from build123d import *

# Parameters (mm, degrees)
SKETCH1_R            = 34.29
BOSS_EXTRUDE1_DEPTH  = 10.16
SKETCH2_R            = 33.02
CUT_EXTRUDE1_DEPTH   = 7.62
SKETCH3_R            = 3.81
BOSS_EXTRUDE2_DEPTH  = 1.27
CUT_EXTRUDE3_REACH   = 51.088
CUT_EXTRUDE4_REACH   = 51.088
CUT_EXTRUDE5_REACH   = 51.546
SKETCH11_R           = 2.032
M2_CLEARANCE_HOLE1_D = 2.4


with BuildPart() as part:
    # Sketch1 → Boss-Extrude1 (new body)
    with BuildSketch(Plane(origin=(0, 0, 0), x_dir=(1, 0, 0), z_dir=(0, 1, 0))):
        with Locations(Location((0, 0, 0), (0, 0, 270))):
            Circle(SKETCH1_R)
    extrude(amount=BOSS_EXTRUDE1_DEPTH)

    # Sketch2 → Cut-Extrude1 (cut)
    with BuildSketch(Plane(origin=(0, 10.16, 0), x_dir=(1, 0, 0), z_dir=(0, 1, 0))):
        with Locations(Location((0, 0, 0), (0, 0, 270))):
            Circle(SKETCH2_R)
    extrude(amount=-CUT_EXTRUDE1_DEPTH, mode=Mode.SUBTRACT)

    # Sketch3 → Boss-Extrude2 (add)
    with BuildSketch(Plane(origin=(0, 2.54, 0), x_dir=(1, 0, 0), z_dir=(0, 1, 0))):
        with Locations(Location((0, -15.24, 0), (0, 0, 270))):
            Circle(SKETCH3_R)
        with Locations(Location((0, 15.24, 0), (0, 0, 270))):
            Circle(SKETCH3_R)
    extrude(amount=BOSS_EXTRUDE2_DEPTH)

    # Sketch8 → Cut-Extrude3 (cut, up to next)
    with BuildSketch(Plane(origin=(0, 2.54, 0), x_dir=(1, 0, 0), z_dir=(0, 1, 0)), mode=Mode.PRIVATE) as cut_extrude3_sk1:
        with BuildLine():
            Line((3.683, 2.032), (-3.683, 2.032))
            ThreePointArc((-3.683, 2.032), (-4.581025612, 1.660025612), (-4.953, 0.762))
            Line((-4.953, 0.762), (-4.953, -0.762))
            ThreePointArc((-4.953, -0.762), (-4.581025612, -1.660025612), (-3.683, -2.032))
            Line((-3.683, -2.032), (3.683, -2.032))
            ThreePointArc((3.683, -2.032), (4.581025612, -1.660025612), (4.953, -0.762))
            Line((4.953, -0.762), (4.953, 0.762))
            ThreePointArc((4.953, 0.762), (4.581025612, 1.660025612), (3.683, 2.032))
        make_face()
    cut_extrude3_tool1 = extrude(cut_extrude3_sk1.sketch, amount=-CUT_EXTRUDE3_REACH, mode=Mode.PRIVATE) & part.part
    add(cut_extrude3_tool1.solids().sort_by_distance((0, 2.54, 0))[0], mode=Mode.SUBTRACT)

    # Sketch9 → Cut-Extrude4 (cut, up to next)
    with BuildSketch(Plane(origin=(0, 2.54, 0), x_dir=(1, 0, 0), z_dir=(0, 1, 0)), mode=Mode.PRIVATE) as cut_extrude4_sk1:
        with BuildLine():
            Line((-12.192, 0), (-9.144, 0))
            ThreePointArc((-9.144, 0), (-8.245974388, 0.371974388), (-7.874, 1.27))
            Line((-7.874, 1.27), (-7.874, 18.796))
            ThreePointArc((-7.874, 18.796), (-8.245974388, 19.694025612), (-9.144, 20.066))
            Line((-9.144, 20.066), (-12.192, 20.066))
            ThreePointArc((-12.192, 20.066), (-13.090025612, 19.694025612), (-13.462, 18.796))
            Line((-13.462, 18.796), (-13.462, 1.27))
            ThreePointArc((-13.462, 1.27), (-13.090025612, 0.371974388), (-12.192, 0))
        make_face()
    cut_extrude4_tool1 = extrude(cut_extrude4_sk1.sketch, amount=-CUT_EXTRUDE4_REACH, mode=Mode.PRIVATE) & part.part
    add(cut_extrude4_tool1.solids().sort_by_distance((-10.668, 2.54, -10.033))[0], mode=Mode.SUBTRACT)

    # Sketch11 → Cut-Extrude5 (cut, up to next)
    with BuildSketch(Plane.XZ, mode=Mode.PRIVATE) as cut_extrude5_sk1:
        with Locations(Location((15.875, 13.843, 0), (0, 0, 270))):
            Circle(SKETCH11_R)
    cut_extrude5_tool1 = extrude(cut_extrude5_sk1.sketch, amount=-CUT_EXTRUDE5_REACH, mode=Mode.PRIVATE) & part.part
    # Sketch11 → Cut-Extrude5 (cut, up to next)
    with BuildSketch(Plane.XZ, mode=Mode.PRIVATE) as cut_extrude5_sk2:
        with Locations(Location((-15.875, 13.843, 0), (0, 0, 270))):
            Circle(SKETCH11_R)
    cut_extrude5_tool2 = extrude(cut_extrude5_sk2.sketch, amount=-CUT_EXTRUDE5_REACH, mode=Mode.PRIVATE) & part.part
    # Sketch11 → Cut-Extrude5 (cut, up to next)
    with BuildSketch(Plane.XZ, mode=Mode.PRIVATE) as cut_extrude5_sk3:
        with Locations(Location((-15.875, -24.257, 0), (0, 0, 270))):
            Circle(SKETCH11_R)
    cut_extrude5_tool3 = extrude(cut_extrude5_sk3.sketch, amount=-CUT_EXTRUDE5_REACH, mode=Mode.PRIVATE) & part.part
    # Sketch11 → Cut-Extrude5 (cut, up to next)
    with BuildSketch(Plane.XZ, mode=Mode.PRIVATE) as cut_extrude5_sk4:
        with Locations(Location((15.875, -24.257, 0), (0, 0, 270))):
            Circle(SKETCH11_R)
    cut_extrude5_tool4 = extrude(cut_extrude5_sk4.sketch, amount=-CUT_EXTRUDE5_REACH, mode=Mode.PRIVATE) & part.part
    add(cut_extrude5_tool1.solids().sort_by_distance((15.875, 0, 13.843))[0], mode=Mode.SUBTRACT)
    add(cut_extrude5_tool2.solids().sort_by_distance((-15.875, 0, 13.843))[0], mode=Mode.SUBTRACT)
    add(cut_extrude5_tool3.solids().sort_by_distance((-15.875, 0, -24.257))[0], mode=Mode.SUBTRACT)
    add(cut_extrude5_tool4.solids().sort_by_distance((15.875, 0, -24.257))[0], mode=Mode.SUBTRACT)

    # M2 Clearance Hole1 (through all)
    with Locations(Plane(origin=(0, 3.81, 0), x_dir=(1, 0, 0), z_dir=(0, 1, 0))):
        with Locations((0, 15.24), (0, -15.24)):
            Hole(M2_CLEARANCE_HOLE1_D / 2)


solid = part.part
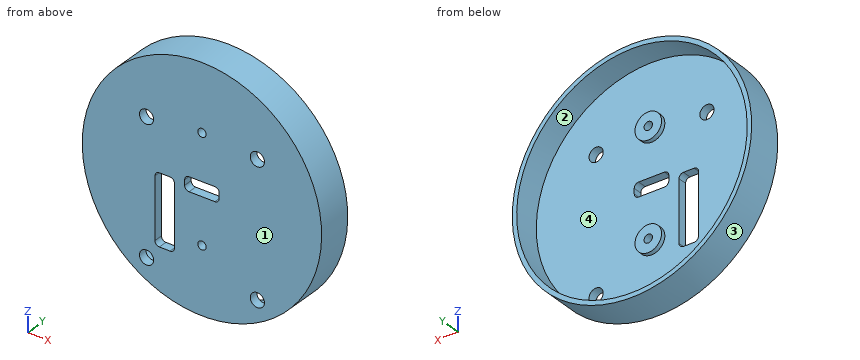
Here's how the part is built. I have some questions about the finished solid (model axes, mm). Face numbers are marked on the shaded views. Coordinates: 2 decimals unless noted, no trailing zeros. Write each loop counter-clockwise with the first axis right and the second up, starting at its lowest first coordinate (ties: lowest second). Pieces come first, ordered by that corner, then holes.
Item 1: I want a section at D-D on y = 5.25. Write out the boundary of the cut face in (x, z).
Item 2: If I drill on line 1 (Z direction, x = 1, y = 9.25); line 2 (X direction, y = 3.05, z = -15.24); line 3 (Y direction, x = -2.5, z = -9.5), over which ranges is the centre line in solid material (lowest first)?
Item 3: I want a section at B-B on z = -15.24. Write out the boundary of the cut face in (x, y).
Item 4: I want a section at A-A on x = 0. Write out the boundary of the cut face in (y, z).
Item 5: If we mould it in two halves opening along X, with no side actions, what happens to the marked faces 1, 2, 3 and 4? For each: +X half, -X half, draft (parallel to the pull), parting line (faces both ways), or undercut.
Item 6: I want a section at C-C on x = 28. Write out the boundary of the cut face in (y, z), and give its area (3 significant figures).
Item 7: Will these pins go through, and if not, where does the flat tip stop? pin 1 (2 mm diameter, centred on x = -1.5, y = 0.5, fed in from -Z); pin 2 (6 mm diameter, centred on y = 5.5, z = -23.5, fed in from -X); pin 3 (0.5 mm diameter, centred on y = 0.5, z = 0, fed in from +X).
Findings below:
1. outline: circle Ø68.58 at (0, 0); hole circle Ø66.04 at (0, 0)
2. line 1: z = -34.28 to -33, 33 to 34.28
2. line 2: x = -30.72 to -29.29, -3.81 to -1.2, 1.2 to 3.81, 29.29 to 30.72
2. line 3: y = 0 to 2.54
3. outline: (-30.72, 0) - (-13.46, 0) - (-13.46, 2.54) - (-29.29, 2.54) - (-29.29, 10.16) - (-30.72, 10.16) - close; (-7.87, 0) - (-1.2, 0) - (-1.2, 3.81) - (-3.81, 3.81) - (-3.81, 2.54) - (-7.87, 2.54) - close; (1.2, 0) - (30.72, 0) - (30.72, 10.16) - (29.29, 10.16) - (29.29, 2.54) - (3.81, 2.54) - (3.81, 3.81) - (1.2, 3.81) - close
4. outline: (0, -34.29) - (10.16, -34.29) - (10.16, -33.02) - (2.54, -33.02) - (2.54, -19.05) - (3.81, -19.05) - (3.81, -16.44) - (0, -16.44) - close; (0, -14.04) - (3.81, -14.04) - (3.81, -11.43) - (2.54, -11.43) - (2.54, -2.03) - (0, -2.03) - close; (0, 2.03) - (2.54, 2.03) - (2.54, 11.43) - (3.81, 11.43) - (3.81, 14.04) - (0, 14.04) - close; (0, 16.44) - (3.81, 16.44) - (3.81, 19.05) - (2.54, 19.05) - (2.54, 33.02) - (10.16, 33.02) - (10.16, 34.29) - (0, 34.29) - close
5. face 1: draft
5. face 2: undercut
5. face 3: parting line
5. face 4: undercut
6. outline: (0, -19.79) - (10.16, -19.79) - (10.16, -17.5) - (2.54, -17.5) - (2.54, 17.5) - (10.16, 17.5) - (10.16, 19.79) - (0, 19.79) - close
6. area: 135 mm2
7. pin 1: stops at z = -34.29
7. pin 2: stops at x = -27.49
7. pin 3: stops at x = 34.29
